Part model, mm, in its own coordinate system. A direction names the side the tool comes from. Round coordinates to 2 decimals unless told otherwise and drop trailing zeros. Order: outer loops, then holes, each group sorted by start corner. A loop starts at its lowest first (then second) coordinate and runs counter-clockwise, first axis right, second up. Notation, with made-up numbers: (64.25, 17) - (70.25, 17) arc R14 cw to (70.25, 33) - close; hole circle Ø6 at (-3.5, -22). An arc over 180 degrees is marked (long way). Answer as a JSON object with one key per item and string values.
```python
from build123d import *

# Parameters (mm, degrees)
F0_R      = 40
F0_R_2    = 35
F1_DEPTH  = 15
F2_R      = 35
F3_DEPTH  = 12
F5_R      = 3
F6_DEPTH  = 42
F7_R      = 5
F8_DEPTH  = 2
F9_R      = 1
F11_W     = 9
F11_H     = 3.350003619
F11_W_2   = 3.350003619
F11_H_2   = 9
F12_DEPTH = 0.5
F13_W     = 30
F13_H     = 2
F14_DEPTH = 12.6
F15_W     = 30
F15_H     = 2
F16_ANGLE = 180


# Not quite as in the source:
# - a fillet or chamfer that OpenCascade refuses, or shapes differently, is made with other operations: its cross-section is extruded or revolved along the edge and cut away or added


with BuildPart() as f1:
    # F0 (on Top) → F1 (new body)
    with BuildSketch(Plane.XY):
        Circle(F0_R)
        Circle(F0_R_2, mode=Mode.SUBTRACT)
    extrude(amount=F1_DEPTH)

    # F2 (on Top) → F3 (join)
    with BuildSketch(Plane.XY):
        Circle(F2_R)
    extrude(amount=F3_DEPTH)

    # F4: fillet of radius 5 on 1 edges, made by hand

    # F4_s1 → F4_t2 (revolve, cut)
    with BuildSketch(Plane.XZ):
        with BuildLine():
            ThreePointArc((39.582575695, 15), (36.8439629074, 14.1833001327), (35, 12))
            Line((35, 12), (35, 15))
            Line((35, 15), (39.582575695, 15))
        make_face()
    revolve(axis=Axis((0, 0, 15), (0, 0, 1)), mode=Mode.SUBTRACT)

    # F5 (on Right) → F6 (join)
    with BuildSketch(Plane.YZ):
        with Locations((0, 7.6651219279)):
            Circle(F5_R)
    extrude(amount=F6_DEPTH)

    # F7 (on face) → F8 (join)
    with BuildSketch(Plane.YZ.offset(42)):
        with Locations((0, 7.6651219279)):
            Circle(F7_R)
    extrude(amount=F8_DEPTH)

    # F9
    f9_edges = [f1.edges().sort_by_distance(p)[0] for p in [
        (44, -5, 7.665122),
    ]]
    fillet(f9_edges, radius=F9_R)

    # F11 (on face) → F12 (join)
    with BuildSketch(Plane.XY.offset(12)):
        with Locations((30.4598965808, 0)):
            Rectangle(F11_W, F11_H)
        with Locations((-30.4598965808, 0)):
            Rectangle(F11_W, F11_H)
        with Locations((0.064526599, 30.4573161602)):
            Rectangle(F11_W_2, F11_H_2)
        with Locations((0.064526599, -30.4573161602)):
            Rectangle(F11_W_2, F11_H_2)
        Polygon((29.9355077939, -18.884427597), (31.6105096033, -15.9832393602), (23.8162809693, -11.4832393602), (22.1412791598, -14.384427597), align=None)
        Polygon((-21.1475788678, 14.4766572205), (-28.9418075019, 18.9766572205), (-30.6168093114, 16.0754689837), (-22.8225806773, 11.5754689837), align=None)
        Polygon((19.4819840184, 29.4502744503), (16.5807957816, 31.1252762598), (12.0807957816, 23.3310476258), (14.9819840184, 21.6560458163), align=None)
        Polygon((-10.9753321418, -23.3033446013), (-13.8765203786, -21.6283427918), (-18.3765203786, -29.4225714259), (-15.4753321418, -31.0975732354), align=None)
        Polygon((31.3365066639, 15.8443492635), (29.6615048544, 18.7455375003), (21.8672762203, 14.2455375003), (23.5422780298, 11.3443492635), align=None)
        Polygon((-23.0965836168, -11.7143590805), (-30.8908122509, -16.2143590805), (-29.2158104414, -19.1155473173), (-21.4215818073, -14.6155473173), align=None)
        Polygon((-15.7493350812, 30.9586831386), (-18.650523318, 29.2836813291), (-14.150523318, 21.489452695), (-11.2493350812, 23.1644545045), align=None)
        Polygon((14.707981079, -21.7949359131), (11.8067928422, -23.4699377226), (16.3067928422, -31.2641663566), (19.207981079, -29.5891645471), align=None)
    extrude(amount=F12_DEPTH)

    # F13 (on face) → F14 (join)
    with BuildSketch(Plane(origin=(0, 0, 0), x_dir=(1, 0, 0), z_dir=(0, 0, -1))):
        with Locations((0, -13.6)):
            Rectangle(F13_W, F13_H)
        with Locations((0, 13.6)):
            Rectangle(F13_W, F13_H)
    extrude(amount=F14_DEPTH)

    # F15 (on face) → F16 (revolve)
    with BuildSketch(Plane(origin=(0, 0, -12.6), x_dir=(1, 0, 0), z_dir=(0, 0, -1))):
        with Locations((0, 13.6)):
            Rectangle(F15_W, F15_H)
    revolve(axis=Axis((9.313e-07, 0, -12.6), (1, 0, 0)), revolution_arc=F16_ANGLE)


solid = f1.part
```
Item 1: Probe L1, parallel to Z at x = 26.5, y = 29; L2, parallel to Z at x = 5.5, y = 29.5; L3, parallel to Y at x = -13.5, z = -11.5. List the from-to ranges inside material, lowest first. Write a range as from..to.
Taken from the geometry:
{"L1": "0..14.99", "L2": "0..12", "L3": "-14.6..-12.6, 12.6..14.6"}
Item 2: Two-plate mould, pull along Y, no slides. Class faces 1 (the flat face through (-26, 15, 12.5)), 2 (the flat face through (0, 14.6, -6)), 3 (the flat face through (-15, -4, -25)), 4 (the cylindrical face through (0.21, -0.321, -27.196)): pulls with the +Y half, pulls with the -Y half, needs draft (parallel to the pull), parting line crosses it, or undercut.
Taken from the geometry:
{"face 1": "undercut", "face 2": "pulls with the +Y half", "face 3": "needs draft", "face 4": "parting line crosses it"}
Item 3: Tool access for faces 5 (the flat face through (14.023, -27.309, 12.246)), 6 (the cylindrical face through (0.21, -0.277, -25.197)), 7 (the flat face through (15, -4, -25)): list every direction of +Z, -Z, +X, -X, +Y, -Y with a clear straight run to the whole face (end or side of a thin tool).
Taken from the geometry:
{"face 5": "+Z", "face 6": "+X, -X", "face 7": "-Z, +X, +Y, -Y"}
Item 4: Cut at A-A (x = 0). Write the cut outline in (y, z), plus the area to 3 significant figures.
Taken from the geometry:
{"outline": "(-40, 0) - (-14.6, 0) - (-14.6, -12.6) arc R14.6 ccw to (14.6, -12.6) - (14.6, 0) - (40, 0) - (40, 15) - (39.58, 15) arc R5 ccw to (35, 12) - (34.96, 12) - (34.96, 12.5) - (25.96, 12.5) - (25.96, 12) - (-25.96, 12) - (-25.96, 12.5) - (-34.96, 12.5) - (-34.96, 12) - (-35, 12) arc R5 ccw to (-39.58, 15) - (-40, 15) - close; hole (-12.6, -12.6) arc R12.6 ccw to (12.6, -12.6) - (12.6, 0) - (-12.6, 0) - close", "area": "1,130 mm2"}
Item 5: Cut at C-C (z = -22). Write the cut outline in (x, y), plus the area to 3 significant figures.
Taken from the geometry:
{"outline": "(-15, -11.17) - (15, -11.17) - (15, -8.39) - (-15, -8.39) - close; (-15, 8.39) - (15, 8.39) - (15, 11.17) - (-15, 11.17) - close", "area": "167 mm2"}
Item 6: Drop flat-ended pins along their axis: P1, Ø1, axis at x = -9.5, y = -22.5, coming from the -Z side; P2, Ø1, axis at x = 15, z = -3, coming from the +Y side; P3, Ø6.5, axis at x = 2.5, z = -4, coming from the -Y side; P4, Ø3, axis at y = -17, z = -13.5, coming from the -X side. Give the stop position or say it passes through.
Taken from the geometry:
{"P1": "z = 0", "P2": "y = 14.6", "P3": "y = -14.6", "P4": "through"}
